Could you check a few things on this model? Use its own coordinates, in mm. Give positions to 0.01 mm unless a question says otherwise; leave off trailing zeros. Order: outer loops, then holes, each group sorted by start corner. A loop starts at its lowest first (then second) coordinate and runs counter-clockwise, first axis right, second up. Notation, with made-up numbers: (-30.5, 70) - (-23.5, 70) arc R31 ccw to (-23.5, 107) - close; hole circle Ø4 at (27.5, 30). An arc over 180 degrees is marked (long way). One line per question, with ' | ' between items. Start each with the question number.
1. Imagine slicing it at D-D (x = 58.5). Please give me the cut outline in (y, z), and give its area (3 significant figures).
2. Imagine slicing it at B-B (x = 0). Please give me the cut outline in (y, z) (3 decimals), and give its area (3 significant figures).
3. If we mould it in two halves opening along Y, with no side actions, what happens to faces 1 (the flat face through (75, -171.45, 43)), 2 (the flat face through (-47, -196.85, -73)), 3 (the flat face through (-47, 196.85, -73)), 4 (the flat face through (-74.4, 171.45, 43.3))? For each: released by +Y, released by -Y, zero draft, split by the parting line, or undercut.
4. Imagine slicing it at A-A (z = 0). Please give me the cut outline in (x, y) (3 decimals).
5. Imagine slicing it at C-C (y = 58.5). Please give me the cut outline in (x, z) (3 decimals).
6. For P1, Ø3.5, axis at y = -79, z = -60, coming from the +X side; P2, Ø21, axis at x = 49, z = 46, coming from the -Y side; P3, Ø1, axis at x = -19.5, y = -118, coming from the +Z side; P4, Ø4, axis at y = 4, z = -37.5, coming from the -X side, each with a flat end and sliding along its axis, tell me the tip position at first contact or that it passes through.
7. I need wall thicknesses on probe 1 along Y at (x, z) = (50.5, 72.5); probe 2 along Z at (x, y) = (0, 19) (3 decimals); probe 3 along X at (y, z) = (179, -51.5). Which ranges of each line are inside material? Lowest first, please. Write a range as from..to.
```python
from build123d import *

# Parameters (mm, degrees)
SKETCH1_R           = 88.9
SKETCH1_R_2         = 85.725
BOSS_EXTRUDE1_DEPTH = 196.85
CUT_EXTRUDE1_START  = -88.9
SKETCH2_W           = 127
SKETCH2_H           = 342.9
CUT_EXTRUDE1_DEPTH  = 31.310716
CIRPATTERN1_COUNT   = 3


with BuildPart() as part:
    # Sketch1 → Boss-Extrude1 (new body, symmetric)
    with BuildSketch(Plane(origin=(0, 0, 0), x_dir=(1, 0, 0), z_dir=(0, 1, 0))):
        Circle(SKETCH1_R)
        Circle(SKETCH1_R_2, mode=Mode.SUBTRACT)
    extrude(amount=BOSS_EXTRUDE1_DEPTH, both=True)

    # Sketch2 → Cut-Extrude1 (cut)
    with BuildSketch(Plane.XY.offset(CUT_EXTRUDE1_START)):
        Rectangle(SKETCH2_W, SKETCH2_H)
    cut_extrude1 = extrude(amount=CUT_EXTRUDE1_DEPTH, mode=Mode.SUBTRACT)

    # CirPattern1: Cut-Extrude1 ×3 about axis
    cirpattern1_axis = Axis((0, 0, 0), (0, 1, 0))
    for i in range(1, CIRPATTERN1_COUNT):
        add(cut_extrude1.rotate(cirpattern1_axis, i * 360 / CIRPATTERN1_COUNT), mode=Mode.SUBTRACT)


solid = part.part
```
Results found:
1) outline: (-196.85, -66.94) - (-171.45, -66.94) - (-171.45, -62.66) - (-196.85, -62.66) - close; (-196.85, 62.66) - (-171.45, 62.66) - (-171.45, 66.94) - (-196.85, 66.94) - close; (171.45, -66.94) - (196.85, -66.94) - (196.85, -62.66) - (171.45, -62.66) - close; (171.45, 62.66) - (196.85, 62.66) - (196.85, 66.94) - (171.45, 66.94) - close | area: 435 mm2
2) outline: (-196.85, -88.9) - (-171.45, -88.9) - (-171.45, -85.725) - (-196.85, -85.725) - close; (-196.85, 85.725) - (196.85, 85.725) - (196.85, 88.9) - (-196.85, 88.9) - close; (171.45, -88.9) - (196.85, -88.9) - (196.85, -85.725) - (171.45, -85.725) - close | area: 1,410 mm2
3) face 1: undercut | face 2: released by -Y | face 3: released by +Y | face 4: undercut
4) outline: (-88.9, -196.85) - (-85.725, -196.85) - (-85.725, -171.45) - (-88.9, -171.45) - close; (-88.9, 171.45) - (-85.725, 171.45) - (-85.725, 196.85) - (-88.9, 196.85) - close; (85.725, -196.85) - (88.9, -196.85) - (88.9, -171.45) - (85.725, -171.45) - close; (85.725, 171.45) - (88.9, 171.45) - (88.9, 196.85) - (85.725, 196.85) - close
5) outline: (-85.632, -23.884) arc R88.9 ccw to (-63.5, -62.217) - (-63.5, -57.589) arc R85.725 cw to (-81.624, -26.198) - close; (-22.132, 86.101) - (-18.124, 83.787) arc R85.725 cw to (18.124, 83.787) - (22.132, 86.101) arc R88.9 ccw to start; (63.5, -62.217) arc R88.9 ccw to (85.632, -23.884) - (81.624, -26.198) arc R85.725 cw to (63.5, -57.589) - close
6) P1: stops at x = 67.16 | P2: passes through | P3: stops at z = 86.85 | P4: stops at x = -81.5
7) probe 1: y = -196.85..-171.45, 171.45..196.85 | probe 2: z = 85.725..88.9 | probe 3: x = -72.46..-68.53, 68.53..72.46
